Verification items for the finished model (mm, model axes). A direction names the side the tool comes from. Give positions to 0.01 mm unless a question says otherwise; leave off trailing zeros. Loops run counter-clockwise (first coordinate to the right, second up) from the corner with the lowest first, then second, coordinate; pieces in that order, holes last. Notation, with made-up numbers: (54, -38.5) - (62, -38.5) arc R26 cw to (62, -17.5) - close; hole circle Ø1 at (18.25, -28.5). An arc over 180 degrees is marked (long way). Answer in a Markdown table with one row per item.
```python
from build123d import *

# Parameters (mm, degrees)
BOSS_EXTRUDE1_DEPTH = 24
SKETCH5_R           = 6.5
BOSS_EXTRUDE3_DEPTH = 29.899298
SKETCH3_R           = 3
CUT_EXTRUDE1_DEPTH  = 30.899298428
FILLET1_R           = 3
CHAMFER1_SIZE       = 1


with BuildPart() as part:
    # Sketch1 → Boss-Extrude1 (new body)
    with BuildSketch(Plane.XY):
        Polygon((0, 15), (14.899298428, 15), (14.899298428, -14.949649214), (-15, -14.949649214), (-15, 15), align=None)
        Polygon((-9.966432809, 9.966432809), (-4.741432809, 9.966432809), (-3.1, 8.307461143), (-5.5, 8.307461143), (-5.5, 6.667461143), (-2.79, 3.957461143), (2.79, 3.957461143), (5.5, 6.667461143), (5.5, 8.307461143), (3.1, 8.307461143), (4.741432809, 9.966432809), (9.966432809, 9.966432809), (9.966432809, 4.741432809), (8.307461143, 3.1), (8.307461143, 5.5), (6.667461143, 5.5), (3.957461143, 2.79), (3.957461143, -2.79), (6.667461143, -5.5), (8.307461143, -5.5), (8.307461143, -3.1), (9.966432809, -4.741432809), (9.966432809, -9.966432809), (4.741432809, -9.966432809), (3.1, -8.307461143), (5.5, -8.307461143), (5.5, -6.667461143), (2.79, -3.957461143), (-2.79, -3.957461143), (-5.5, -6.667461143), (-5.5, -8.307461143), (-3.1, -8.307461143), (-4.741432809, -9.966432809), (-9.966432809, -9.966432809), (-9.966432809, -4.741432809), (-8.307461143, -3.1), (-8.307461143, -5.5), (-6.667461143, -5.5), (-3.957461143, -2.79), (-3.957461143, 2.79), (-6.667461143, 5.5), (-8.307461143, 5.5), (-8.307461143, 3.1), (-9.966432809, 4.741432809), align=None, mode=Mode.SUBTRACT)
    extrude(amount=BOSS_EXTRUDE1_DEPTH)

    # Sketch5 → Boss-Extrude3 (add, through all)
    with BuildSketch(Plane.ZY.offset(15)):
        with BuildLine():
            Line((0, 15), (0, 22.5))
            Line((0, 22.5), (0, 29))
            ThreePointArc((0, 29), (12, 41), (24, 29))
            Line((24, 29), (24, 22.5))
            Line((24, 22.5), (24, 15))
            Line((24, 15), (0, 15))
        make_face()
        with Locations((12, 29)):
            Circle(SKETCH5_R, mode=Mode.SUBTRACT)
    extrude(amount=-BOSS_EXTRUDE3_DEPTH)

    # Sketch3 → Cut-Extrude1 (cut, through all)
    with BuildSketch(Plane.ZY.offset(15)):
        with Locations((12, 0)):
            Circle(SKETCH3_R)
    extrude(amount=-CUT_EXTRUDE1_DEPTH, mode=Mode.SUBTRACT)

    # Fillet1
    fillet1_edges = [part.edges().sort_by_distance(p)[0] for p in [
        (-0.050350786, -14.949649214, 24),
        (14.899298214, 7.025175393, 24),
        (14.899298, 41, 12),
        (-15, 41, 12),
        (14.899298428, 0.025175393, 0),
        (-0.050350786, -14.949649214, 0),
        (-15, 7.025175393, 0),
        (-15, 7.025175393, 24),
        (14.899298428, -14.949649214, 12),
        (-15, -14.949649214, 12),
    ]]
    fillet(fillet1_edges, radius=FILLET1_R)

    # Chamfer1
    chamfer1_edges = [part.edges().sort_by_distance(p)[0] for p in [
        (14.899298, 29, 5.5),
        (-15, 29, 5.5),
        (14.899298428, 0, 9),
        (-15, 0, 9),
    ]]
    chamfer(chamfer1_edges, length=CHAMFER1_SIZE)


solid = part.part
```
Q1. Draft check along Z on faces 1 (the face through (0, 8, 0)), 2 (the face through (-0.246, 34.481, 15.494)), 3 (the face through (-3.957, 0, 20)). Enter one of: +Z half, -Z half, draft (parallel to the pull), parting line (faces both ways), or undercut.
Completed:
| item | result |
|---|---|
| face 1 | -Z half |
| face 2 | undercut |
| face 3 | draft |
Q2. Sectioned sample at B-B (y = 0). Record the cut outline in (x, z).
Completed:
| item | result |
|---|---|
| outline | (-15, 3) arc R3 ccw to (-12, 0) - (-3.96, 0) - (-3.96, 9) - (-14, 9) - (-15, 8) - close; (-15, 16) - (-14, 15) - (-3.96, 15) - (-3.96, 24) - (-12, 24) arc R3 ccw to (-15, 21) - close; (3.96, 0) - (11.9, 0) arc R3 ccw to (14.9, 3) - (14.9, 8) - (13.9, 9) - (3.96, 9) - close; (3.96, 15) - (13.9, 15) - (14.9, 16) - (14.9, 21) arc R3 ccw to (11.9, 24) - (3.96, 24) - close |
Q3. Go/stop test with flat-tipped pins: P1, Ø5.5, axis at x = -6.5, z = 16.5, coming from the +Y side; P2, Ø0.7, axis at x = -3.5, z = 8.5, coming from the +Y side; P3, Ø1.5, axis at y = 13.5, z = 2.5, coming from the +X side; P4, Ø3, axis at x = -2.5, y = 32.5, coming from the -Z side. Record where each tip stops, or that it passes through.
Completed:
| item | result |
|---|---|
| P1 | y = 40.87 |
| P2 | y = 40.58 |
| P3 | x = 14.9 |
| P4 | z = 0.17 |
Q4. Sectioned sample at A-A (x = 2). Record the cut outline in (y, z).
Completed:
| item | result |
|---|---|
| outline | (-14.95, 3) arc R3 ccw to (-11.95, 0) - (-3.96, 0) - (-3.96, 24) - (-11.95, 24) arc R3 ccw to (-14.95, 21) - close; (3.96, 0) - (29, 0) arc R12 ccw to (29, 24) - (3.96, 24) - close; hole circle Ø13 at (29, 12) |
Q5. Sectioned sample at C-C (z = 7.25). Give the number of separate pieces and of enclosed holes in the cut face, and give its area (3 significant figures).
Completed:
| item | result |
|---|---|
| separate pieces | 2 |
| enclosed holes | 1 |
| area | 1,180 mm^2 |
Q6. Tool access check on faces 4 (the face through (0, 3.957, 12)), 5 (the face through (-15, 8, 12)). Record the directions out of +Z, -Z, +X, -X, +Y, -Y that give a thin tool (end or side, any length) a straight path to the whole face; none if there is none.
Completed:
| item | result |
|---|---|
| face 4 | +Z, -Z |
| face 5 | +Z, -Z, -X, +Y, -Y |
Q7. Thickness scan on line 1 (X direction, y = 1, z = 17); line 2 (Z direction, x = -6.75, y = 0); line 3 (Y direction, x = 0, z = 12). Record the ranges inside material, lowest first.
Completed:
| item | result |
|---|---|
| line 1 | -15 to -3.96, 3.96 to 14.9 |
| line 2 | 0 to 9, 15 to 24 |
| line 3 | -14.95 to -3.96, 3.96 to 22.5, 35.5 to 41 |
